Geometry check sheet. Reference: drawing and pictorial views, mm from the part's lowest x, y, z. Give positions to 0.01 mm unless a question says otherwise; leave off trailing zeros. Write each loop counter-clockwise with the first axis right and the second up, starting at its lowest first coordinate (ties: lowest second). Pieces come first, ordered by that corner, then holes. Notation, with made-up numbers: M 23,21.25 L 37,21.25 A29 cw 37,59.25 Z; hole C 30.5,-7.75 d11. An arc over 180 degrees is marked long. Answer as a JSON object with one key per item and string values.
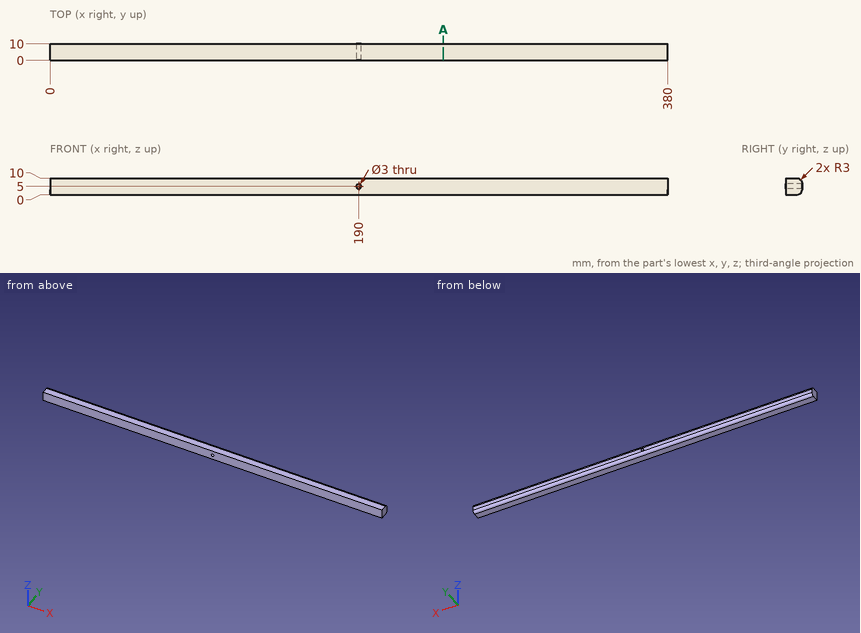
1) Thickness scan on L1, parallel to Z at x = 190, y = 4.75; L2, parallel to Z at x = 93.5, y = 7.5; L3, parallel to Y at x = 83.5, z = 2.75. Record the ranges inside material, lowest first.
Completed:
{"L1": "z = 0 to 3.5, 6.5 to 10", "L2": "z = 0.04 to 9.96", "L3": "y = 0 to 9.99"}
2) Section check A-A on x = 242. Record the boundary of the cut face in (y, z), and give its area (3 significant figures).
Completed:
{"outline": "M 0,0 L 7,0 A3 ccw 10,3 L 10,7 A3 ccw 7,10 L 0,10 Z", "area": "96.1 mm2"}
3) Go/stop test with a flat-tipped pin: pin 1 (1.5 mm diameter, centred on x = 254.5, y = 8, fed in from -Z). Record where the tip stops, or that it passes through.
Completed:
{"pin 1": "stops at z = 0.01"}
